Here's how the part is built. I have some questions about the finished solid (model axes, mm). Give positions to 0.01 mm unless a question says otherwise; leave off trailing zeros. Answer as CSV lines item,"result". Start each with the question number.
Item 1: If I drill on line 1 along Y through (x, z) = (293, 2.55); line 2 along Y through (x, z) = (253, 0.85); line 3 along Y through (x, z) = (5, 2.1), over which ranges is the centre line in solid material (lowest first)? Write a range as from..to.
Item 2: If we mould it in two halves opening along Y, with no side actions, what happens to faces 1 (the flat face through (211, 16, 0)), 2 (the cylindrical face through (399.93, -2.87, 1.48)), 3 (the cylindrical face through (427.99, -0.77, 1.48))? For each: released by +Y, released by -Y, zero draft, split by the parting line, or undercut.
Item 3: I want a section at A-A on z = 1.7. Give the number of separate pieces and of enclosed holes in the cut face, plus the area to 3 significant figures.
from build123d import *

# Parameters (mm, degrees)
SKETCH1_R               = 2
SKETCH1_R_2             = 7.5
SKETCH1_R_3             = 2.5
BOSS_EXTRUDE1_DEPTH     = 3
CUT_EXTRUDE1_DEPTH      = 430.43916915
CUT_EXTRUDE1_DEPTH_BACK = 430.43916915
CUT_EXTRUDE2_DEPTH      = 430.43916915
CUT_EXTRUDE2_DEPTH_BACK = 430.43916915
SKETCH5_R               = 2.5
SKETCH7_R               = 1.5
CUT_EXTRUDE4_DEPTH      = 3
CUT_EXTRUDE6_DEPTH      = 10


with BuildPart() as part:
    # Sketch1 → Boss-Extrude1 (new body)
    with BuildSketch(Plane.XY):
        with BuildLine():
            Line((0, 35), (0, -35))
            Line((0, -35), (393, -35))
            ThreePointArc((393, -35), (428, 0), (393, 35))
            Line((393, 35), (0, 35))
        make_face()
        with Locations((5, 29)):
            Circle(SKETCH1_R, mode=Mode.SUBTRACT)
        with Locations(Location((5, -29, 0), (0, 0, 180))):
            Circle(SKETCH1_R, mode=Mode.SUBTRACT)
        with Locations((393, 0)):
            Circle(SKETCH1_R_2, mode=Mode.SUBTRACT)
        with Locations((103, 0)):
            Circle(SKETCH1_R_3, mode=Mode.SUBTRACT)
        with Locations((31, 29)):
            Circle(SKETCH1_R, mode=Mode.SUBTRACT)
        with Locations((31, -29)):
            Circle(SKETCH1_R, mode=Mode.SUBTRACT)
        with Locations((5, 0)):
            Circle(SKETCH1_R, mode=Mode.SUBTRACT)
    extrude(amount=BOSS_EXTRUDE1_DEPTH)

    # Sketch4 → Cut-Extrude1 (cut, two sides: drawn at the far end of the back side and taken through both)
    with BuildSketch(Plane.XY.offset(3).offset(-CUT_EXTRUDE1_DEPTH_BACK)):
        with BuildLine():
            Line((55.5, 27), (55.5, 12))
            ThreePointArc((55.5, 12), (53, 9.5), (50.5, 12))
            Line((50.5, 12), (50.5, 27))
            ThreePointArc((50.5, 27), (53, 29.5), (55.5, 27))
        make_face()
        with BuildLine():
            Line((155.5, 22), (155.5, 7))
            ThreePointArc((155.5, 7), (153, 4.5), (150.5, 7))
            Line((150.5, 7), (150.5, 22))
            ThreePointArc((150.5, 22), (153, 24.5), (155.5, 22))
        make_face()
        with BuildLine():
            Line((155.5, -22), (155.5, -7))
            ThreePointArc((155.5, -7), (153, -4.5), (150.5, -7))
            Line((150.5, -7), (150.5, -22))
            ThreePointArc((150.5, -22), (153, -24.5), (155.5, -22))
        make_face()
        with BuildLine():
            Line((55.5, -27), (55.5, -12))
            ThreePointArc((55.5, -12), (53, -9.5), (50.5, -12))
            Line((50.5, -12), (50.5, -27))
            ThreePointArc((50.5, -27), (53, -29.5), (55.5, -27))
        make_face()
    extrude(amount=CUT_EXTRUDE1_DEPTH + CUT_EXTRUDE1_DEPTH_BACK, mode=Mode.SUBTRACT)

    # Sketch5 → Cut-Extrude2 (cut, two sides: drawn at the far end of the back side and taken through both)
    with BuildSketch(Plane.XY.offset(3).offset(-CUT_EXTRUDE2_DEPTH_BACK)):
        with Locations((335.5, 0)):
            Circle(SKETCH5_R)
    extrude(amount=CUT_EXTRUDE2_DEPTH + CUT_EXTRUDE2_DEPTH_BACK, mode=Mode.SUBTRACT)

    # Sketch7 → Cut-Extrude4 (cut)
    with BuildSketch(Plane.XY.offset(3)):
        with Locations((73, -29)):
            Circle(SKETCH7_R)
        with Locations((133, -29)):
            Circle(SKETCH7_R)
        with Locations((193, -29)):
            Circle(SKETCH7_R)
        with Locations((253, -29)):
            Circle(SKETCH7_R)
        with Locations((313, -29)):
            Circle(SKETCH7_R)
        with Locations((358, -29)):
            Circle(SKETCH7_R)
    extrude(amount=-CUT_EXTRUDE4_DEPTH, mode=Mode.SUBTRACT)

    # Sketch9 → Cut-Extrude6 (cut)
    with BuildSketch(Plane.XY.offset(3)):
        Polygon((223.795, 0), (218.021497308, 10), (206.474491924, 10), (200.700989232, 0), (206.474491924, -10), (218.021497308, -10), align=None)
        Polygon((191.795, 0), (186.021497308, 10), (174.474491924, 10), (168.700989232, 0), (174.474491924, -10), (186.021497308, -10), align=None)
        Polygon((255.795, 0), (250.021497308, 10), (238.474491924, 10), (232.700989232, 0), (238.474491924, -10), (250.021497308, -10), align=None)
        Polygon((287.795, 0), (282.021497308, 10), (270.474491924, 10), (264.700989232, 0), (270.474491924, -10), (282.021497308, -10), align=None)
        Polygon((233.865777575, 16), (231.056886095, 20.865142755), (225.439103137, 20.865142755), (222.630211658, 16), (225.439103137, 11.134857245), (231.056886095, 11.134857245), align=None)
        Polygon((201.865777575, 16), (199.056886095, 20.865142755), (193.439103137, 20.865142755), (190.630211658, 16), (193.439103137, 11.134857245), (199.056886095, 11.134857245), align=None)
        Polygon((265.865777575, 16), (263.056886095, 20.865142755), (257.439103137, 20.865142755), (254.630211658, 16), (257.439103137, 11.134857245), (263.056886095, 11.134857245), align=None)
        Polygon((319.795, 0), (314.021497308, 10), (302.474491924, 10), (296.700989232, 0), (302.474491924, -10), (314.021497308, -10), align=None)
        Polygon((297.865777575, 16), (295.056886095, 20.865142755), (289.439103137, 20.865142755), (286.630211658, 16), (289.439103137, 11.134857245), (295.056886095, 11.134857245), align=None)
        Polygon((295.056886095, -11.134857245), (297.865777575, -16), (295.056886095, -20.865142755), (289.439103137, -20.865142755), (286.630211658, -16), (289.439103137, -11.134857245), align=None)
        Polygon((263.056886095, -11.134857245), (265.865777575, -16), (263.056886095, -20.865142755), (257.439103137, -20.865142755), (254.630211658, -16), (257.439103137, -11.134857245), align=None)
        Polygon((231.056886095, -11.134857245), (233.865777575, -16), (231.056886095, -20.865142755), (225.439103137, -20.865142755), (222.630211658, -16), (225.439103137, -11.134857245), align=None)
        Polygon((199.056886095, -11.134857245), (201.865777575, -16), (199.056886095, -20.865142755), (193.439103137, -20.865142755), (190.630211658, -16), (193.439103137, -11.134857245), align=None)
    extrude(amount=-CUT_EXTRUDE6_DEPTH, mode=Mode.SUBTRACT)


solid = part.part
Result:
1,line 1,"-35..-20.87, -11.13..11.13, 20.87..35"
1,line 2,"-35..-30.5, -27.5..-4.84, 4.84..35"
1,line 3,"-35..-31, -27..-2, 2..27, 31..35"
2,face 1,"zero draft"
2,face 2,"undercut"
2,face 3,"split by the parting line"
3,separate pieces,"1"
3,enclosed holes,"31"
3,area,"26,300 mm^2"
